Input: part model. Units: mm. Frame: model coordinates. Face numbers are marked on the shaded views. A direction names the side the tool comes from. Give positions to 0.01 mm unless a question says otherwise; leave off trailing zeros. Write each loop counter-clockwise with the first axis right and the second up, starting at its lowest first coordinate (ties: lowest second). Pieces come first, ordered by that corner, then holes. Notation, with made-up numbers: (39, 56.5) - (48, 56.5) arc R27 cw to (48, 95.5) - close; hole circle Ø11 at (-7.75, 89). An arc over 180 degrees is marked (long way). Answer as CSV lines item,"result".
```python
from build123d import *

# Parameters (mm, degrees)
SKETCH_W     = 200
SKETCH_H     = 200
PAD_DEPTH    = 10
SKETCH001_R  = 30
SKETCH001_W  = 42.426406
SKETCH001_H  = 42.426406
POCKET_DEPTH = 5


with BuildPart() as part:
    # Sketch → Pad (new body)
    with BuildSketch(Plane.XY):
        Rectangle(SKETCH_W, SKETCH_H)
    extrude(amount=PAD_DEPTH)

    # Sketch001 (on Face6 of Pad) → Pocket (cut)
    with BuildSketch(Plane.XY.offset(10)):
        with Locations((50, 50)):
            Circle(SKETCH001_R)
        with BuildLine():
            add(Edge.make_bspline(
                [(-28.786797, -71.213203), (-10.415623, -52.84203), (-51.421015, -30.207812), (-92.426407, -7.573593), (-69.792188, -48.578985), (-47.15797, -89.584377), (-28.786797, -71.213203)],
                knots=[0, 0, 0, 2.094395, 2.094395, 4.18879, 4.18879, 6.283185, 6.283185, 6.283185], degree=2, weights=[1, 0.5, 1, 0.5, 1, 0.5, 1]))
        make_face()
        Polygon((75.980762, -65), (50, -20), (24.019238, -65), align=None)
        with Locations((-50, 50)):
            Rectangle(SKETCH001_W, SKETCH001_H)
    extrude(amount=-POCKET_DEPTH, mode=Mode.SUBTRACT)


solid = part.part
```
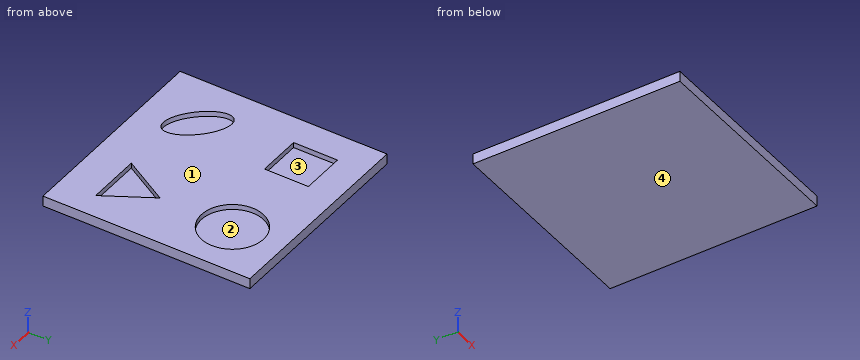
Item 1: Cut plane A-A on y = 50. Return the cut outline in (x, z).
The answers:
outline,"(-100, 0) - (100, 0) - (100, 10) - (80, 10) - (80, 5) - (20, 5) - (20, 10) - (-28.79, 10) - (-28.79, 5) - (-71.21, 5) - (-71.21, 10) - (-100, 10) - close"
Item 2: Mould query, pull axis X, two halves, no side actions, for the marked faces 3 and 4. Classes: +X half, -X half, draft (parallel to the pull), parting line (faces both ways), or undercut.
The answers:
face 3,"undercut"
face 4,"draft"
Item 3: Cut plane C-C on x = 30. Return the cut outline in (y, z), plus the area to 3 significant figures.
The answers:
outline,"(-100, 0) - (100, 0) - (100, 10) - (72.36, 10) - (72.36, 5) - (27.64, 5) - (27.64, 10) - (-54.64, 10) - (-54.64, 5) - (-65, 5) - (-65, 10) - (-100, 10) - close"
area,"1,720 mm²"
Item 4: Ray query, line 1 (Y direction, x = 50, z = 8.95); line 2 (Y direction, x = 25, z = 6.5); line 3 (X direction, y = -52.5, z = 9). Return the intervals inside material, ascending. Write a range as from..to.
The answers:
line 1,"-100..-65, -20..20, 80..100"
line 2,"-100..-65, -63.3..33.42, 66.58..100"
line 3,"-100..-67.37, -29.63..31.24, 68.76..100"
Item 5: Reachability of the marked faces 1 and 2 from +Z, -Z, +X, -X, +Y, -Y: full face, straight path, thin tool, end or side. Return the list, or none.
The answers:
face 1,"+Z, +X, -X, +Y, -Y"
face 2,"+Z"
Item 6: Contact query for flat-ended pins moving along their axis: pin 1 (21 mm diameter, centred on x = -51, y = 45.5, fed in from +Z); pin 2 (4 mm diameter, centred on x = -79, y = 73, fed in from -Z). Output: stop coordinate, or through.
The answers:
pin 1,"z = 5"
pin 2,"z = 0"
Item 7: Cut plane B-B on z = 7.5. Count the separate pieces of the cut face and the enclosed holes in it, plus the area to 3 significant figures.
The answers:
separate pieces,"1"
enclosed holes,"4"
area,"32,800 mm²"
